Here's how the part is built. I have some questions about the finished solid (model axes, mm). A direction names the side the tool comes from. Round coordinates to 2 decimals unless told otherwise and drop trailing zeros. Loops run counter-clockwise (first coordinate to the right, second up) from the corner with the lowest first, then second, coordinate; pieces in that order, holes last. Notation, with made-up numbers: M 60.5,51 L 118.5,51 A27 ccw 118.5,68 Z; hole C 31.5,0 d1. An arc over 180 degrees is marked long. Use a Markdown table: item, result.
Autodesk Inventor part; units mm, degrees
ref_plane "YZ Plane" through (0, 0, 0) normal (1, 0, 0) x (0, 1, 0)
ref_plane "XZ Plane" through (0, 0, 0) normal (0, 1, 0) x (-1, 0, 0)
ref_plane "XY Plane" through (0, 0, 0) normal (0, 0, 1) x (1, 0, 0)
sketch "Sketch1" plane through (0, 0, 0) normal (0, 0, 1) x (1, 0, 0)
  line L0 (-12.7, -25.4) -> (12.7, -25.4)
  line L1 (12.7, -25.4) -> (12.7, 25.4)
  line L2 (12.7, 25.4) -> (-12.7, 25.4)
  line L3 (-12.7, 25.4) -> (-12.7, -25.4)
  line L4 (-12.7, -25.4) -> (12.7, 25.4) construction
  line L5 (12.7, -25.4) -> (-12.7, 25.4) construction
  line L6 (-11.1125, 23.8125) -> (11.1125, 23.8125)
  line L7 (11.1125, 23.8125) -> (11.1125, -23.8125)
  line L8 (11.1125, -23.8125) -> (-11.1125, -23.8125)
  line L9 (-11.1125, -23.8125) -> (-11.1125, 23.8125)
  point P0 (0, 0)
  dimension "width" = 25.4
  dimension "height" = 50.8
  dimension "thickness" = 1.5875
extrude "Extrusion1" add sketch "Sketch1" along normal mid plane 120.65
sketch "Sketch2" plane through (-12.7, -25.4, 60.325) normal (-1, 0, 0) x (0, 0, 1)
  circle A0 centre (-70.485, 25.4) radius 31.75 construction
  line L0 (-120.65, 0) -> (-120.65, 50.8)
  line L1 (-60.325, 50.8) -> (-60.325, 0) construction
  line L2 (0, 0) -> (-120.65, 0) construction
  line L3 (-120.65, 50.8) -> (0, 50.8) construction
  circle A1 centre (-70.485, 25.4) radius 19.05
  point P0 (-107.95, 38.1)
  point P1 (-107.95, 25.4)
  point P2 (-107.95, 12.7)
  point P3 (-12.7, 38.1)
  point P4 (-12.7, 25.4)
  point P5 (-12.7, 12.7)
  point P6 (-70.485, 57.15)
  point P7 (-60.325, 25.4)
  point P8 (-97.9813, 41.275)
  point P9 (-97.9813, 9.525)
  point P10 (-70.485, -6.35)
  point P11 (-42.9887, 9.525)
  point P12 (-42.9887, 41.275)
  dimension "d5" = 63.5
  dimension "d17" = 12.7
  dimension "d18" = 12.7
  dimension "d19" = 12.7
  dimension "d23" = 10.16
  dimension "d26" = 360
  dimension "d28" = 38.1
hole "Hole1" at (-12.7, 12.7, -47.625) at (-12.7, 0, -47.625) at (-12.7, -12.7, -47.625) at (-12.7, -12.7, 47.625) at (-12.7, 0, 47.625) at (-12.7, 12.7, 47.625) at (-12.7, 15.875, 17.3363) at (-12.7, -15.875, 17.3363) at (-12.7, -15.875, -37.6563) at (-12.7, 15.875, -37.6563) direction (1, 0, 0) diameter 5.1054 end through all
extrude "Extrusion3" cut sketch "Sketch2" against normal through all
sketch "Sketch4" plane through (-12.7, 25.4, 60.325) normal (0, 1, 0) x (1, 0, 0)
  line L0 (18.415, 34.925) -> (18.415, 85.725) construction
  line L1 (25.4, 0) -> (0, 0) construction
  line L2 (0, 120.65) -> (0, 0) construction
  point P0 (18.415, 60.325)
  point P1 (12.7, 0)
  point P2 (0, 60.325)
  dimension "d41" = 50.8
  dimension "d42" = 18.415
hole "Hole2" at (5.715, 25.4, -25.4) at (5.715, 25.4, 25.4) direction (0, -1, 0) diameter 5.1054 end through all
properties part number "GP5-001" material "Aluminum 6061"
1. Which directions (+Z, -Z, +X, -X, +Y, -Y) give clear straight access to the entire face, cutting with the end or side of a thin tool? Please do faces 4 (the face through (11.917, -11.147, 45.599)), 5 (the face through (11.112, 0, 13)).
Answer sheet:
| item | result |
|---|---|
| face 4 | +X, -X |
| face 5 | +Z, -Z |
2. Imagine slicing it at A-A, the plane z = -25.4. Write out the boundary of the cut face in (x, y), then the cut area to 3 significant figures.
Answer sheet:
| item | result |
|---|---|
| outline | M -12.7,-25.4 L 3.16,-25.4 L 3.16,-23.81 L -11.11,-23.81 L -11.11,-11.43 L -12.7,-11.43 Z; M -12.7,11.43 L -11.11,11.43 L -11.11,23.81 L 3.16,23.81 L 3.16,25.4 L -12.7,25.4 Z; M 8.27,-25.4 L 12.7,-25.4 L 12.7,-11.43 L 11.11,-11.43 L 11.11,-23.81 L 8.27,-23.81 Z; M 8.27,23.81 L 11.11,23.81 L 11.11,11.43 L 12.7,11.43 L 12.7,25.4 L 8.27,25.4 Z |
| area | 143 mm2 |
3. We'd pull the mould along Z, two halves only. Please class faces 1 (the face through (-11.895, -0.112, 45.075)), 2 (the face through (0, -23.812, -1)), 3 (the face through (-11.3, 2, -60.325)): +Z half, -Z half, draft (parallel to the pull), parting line (faces both ways), or undercut.
Answer sheet:
| item | result |
|---|---|
| face 1 | undercut |
| face 2 | draft |
| face 3 | -Z half |
4. Imagine slicing it at C-C, the plane z = -10.16. Write out the boundary of the cut face in (x, y).
Answer sheet:
| item | result |
|---|---|
| outline | M -12.7,-25.4 L 12.7,-25.4 L 12.7,-19.05 L 11.11,-19.05 L 11.11,-23.81 L -11.11,-23.81 L -11.11,-19.05 L -12.7,-19.05 Z; M -12.7,19.05 L -11.11,19.05 L -11.11,23.81 L 11.11,23.81 L 11.11,19.05 L 12.7,19.05 L 12.7,25.4 L -12.7,25.4 Z |
5. I need wall thicknesses on probe 1 along Y at (x, z) = (7.5, -22); probe 2 along X at (y, z) = (-1, -39); probe 3 along Z at (x, y) = (11.7, 12.7) (3 decimals). Which ranges of each line are inside material? Lowest first, please. Write a range as from..to.
Answer sheet:
| item | result |
|---|---|
| probe 1 | -25.4..-23.81, 23.81..25.4 |
| probe 2 | -12.7..-11.11, 11.11..12.7 |
| probe 3 | -60.325..-50.178, -45.072..-24.359, 4.039..45.072, 50.178..60.325 |
6. Imagine slicing it at B-B, the plane y = 22.5. Write out the boundary of the cut face in (x, z) (1 decimal).
Answer sheet:
| item | result |
|---|---|
| outline | M -12.7,-60.3 L -11.1,-60.3 L -11.1,60.3 L -12.7,60.3 Z; M 11.1,-60.3 L 12.7,-60.3 L 12.7,60.3 L 11.1,60.3 Z |
7. Imagine slicing it at D-D, the plane x = -1.5. Write out the boundary of the cut face in (y, z) (1 decimal).
Answer sheet:
| item | result |
|---|---|
| outline | M -25.4,-60.3 L -23.8,-60.3 L -23.8,60.3 L -25.4,60.3 Z; M 23.8,-60.3 L 25.4,-60.3 L 25.4,60.3 L 23.8,60.3 Z |
